```python
from build123d import *

# Parameters (mm, degrees)
REVOLUTION_ANGLE = 90
SKETCH001_W      = 30
SKETCH001_H      = 18.068252
PAD_DEPTH        = 5
SKETCH002_R      = 9.75
POCKET_DEPTH     = 5
FILLET_R         = 13
FILLET001_R      = 13


with BuildPart() as part:
    # Sketch → Revolution (revolve, symmetric)
    with BuildSketch(Plane.XY) as revolution_sk:
        with BuildLine():
            ThreePointArc((27.507267, 229.338864), (0, 255), (-27.507267, 229.338864))
            Line((-36.5, 100), (-27.507267, 229.338864))
            Line((-36.5, 100), (-32.5, 100))
            Line((-32.5, 100), (-22.5, 229.239629))
            ThreePointArc((22.5, 229.239629), (0, 250.06593), (-22.5, 229.239629))
            Line((22.5, 229.239629), (32.5, 100))
            Line((32.5, 100), (36.5, 100))
            Line((36.5, 100), (27.507267, 229.338864))
        make_face()
    revolve(axis=Axis((0, 0, 0), (1, 0, 0)), revolution_arc=REVOLUTION_ANGLE / 2)
    revolve(revolution_sk.sketch, axis=Axis((0, 0, 0), (-1, 0, 0)), revolution_arc=REVOLUTION_ANGLE / 2)

    # Sketch001 (on Face1 of CopyFusion) → Pad (new body)
    with BuildSketch(Plane(origin=(0, 0, 0), x_dir=(1, 0, 0), z_dir=(0, -0.707107, 0.707107))):
        with Locations((0, 259.214452)):
            Rectangle(SKETCH001_W, SKETCH001_H)
    extrude(amount=-PAD_DEPTH)

    # Sketch002 (on Face15 of Pad) → Pocket (cut)
    with BuildSketch(Plane(origin=(0, 0, 0), x_dir=(1, 0, 0), z_dir=(0, -0.707107, 0.707107))):
        with Locations((0, 272.75)):
            Circle(SKETCH002_R)
    extrude(amount=-POCKET_DEPTH, mode=Mode.SUBTRACT)

    # Fillet
    fillet_edges = [part.edges().sort_by_distance(p)[0] for p in [
        (-34.5, 70.710678, -70.710678),
        (34.5, 70.710678, -70.710678),
    ]]
    fillet(fillet_edges, radius=FILLET_R)

    # Fillet001
    fillet001_edges = [part.edges().sort_by_distance(p)[0] for p in [
        (-34.5, 70.710678, 70.710678),
        (34.5, 70.710678, 70.710678),
    ]]
    fillet(fillet001_edges, radius=FILLET001_R)


solid = part.part
```
Source: CAD feature listing. Evaluate the final solid. Frame: model axes, mm. A direction names the side the tool comes from. Give positions to 0.01 mm unless a question says otherwise; leave off trailing zeros. Write each loop counter-clockwise with the first axis right and the second up, starting at its lowest first coordinate (ties: lowest second). Pieces come first, ordered by that corner, then holes.
1. Pull-direction query (X, two-part tool) for faces 4 (the face through (32.94, 151.19, 1.66)), 5 (the face through (-32.94, 151.19, 1.66)), 6 (the face through (-28.54, 151.16, 1.66)), 7 (the face through (-24, 151, 151)); classes: +X half, -X half, draft (parallel to the pull), parting line (faces both ways), or undercut.
2. Section query A-A (x = -18.5). Return the cut outline in (y, z).
3. First-contact query: pin 1 (8 mm diameter, centred on y = 183.5, z = 181.5, fed in from -X); pin 2 (4 mm diameter, centred on x = 1.5, y = 189, fed in from -Z); pin 3 (5 mm diameter, centred on x = 17.5, z = 73.5, fed in from -Y). Flat tips, straight axial feed; report the tip coordinate or a pass-through.
4. Material intervals for line 1 along Z through (x, y) = (13.5, 184); line 2 along X through (y, z) = (225, -43.5); line 3 along X through (y, z) = (137, -90), sorted ascending.
5. Access query for faces 1 (the face through (15, 185, 182)), 2 (the face through (-15, 185, 182)), 3 (the face through (28.68, 149.35, 1.64)). Directions: +Z, -Z, +X, -X, +Y, -Y. A direction counts if a zero-diameter tool reaches every point of the face in a straight line with its end or side. Return the directions, or none.
Output values:
1. face 4: +X half
1. face 5: -X half
1. face 6: undercut
1. face 7: draft
2. outline: (170, -170) - (175.27, -175.27) arc R247.87 ccw to (175.27, 175.27) - (170, 170) arc R240.42 cw to start
3. pin 1: stops at x = -15
3. pin 2: stops at z = -173.31
3. pin 3: stops at y = 226.25
4. line 1: z = -171.41 to -162.65, 162.65 to 171.41, 176.93 to 184
4. line 2: x = -27.52 to -22.51, 22.51 to 27.52
4. line 3: x = -32.06 to -27.55, 27.55 to 32.06
5. face 1: +Z, +X, +Y
5. face 2: +Z, -X, +Y
5. face 3: -Y
